For this review, use the dimensioned drawing (mm, ordinates from the lowest corner) and the shaded views. A direction names the side the tool comes from. Coordinates: 2 decimals unless noted, no trailing zeros. Order: outer loops, then holes, each group sorted by start corner. A loop starts at its lowest first (then second) coordinate and runs counter-clockwise, first axis right, second up. Notation, with made-up numbers: M 1,-10.5 L 28,-10.5 A23 cw 28,5.5 Z; hole C 71.25,70 d4. An arc over 180 degrees is marked long. Answer in a Markdown table with one row per item.
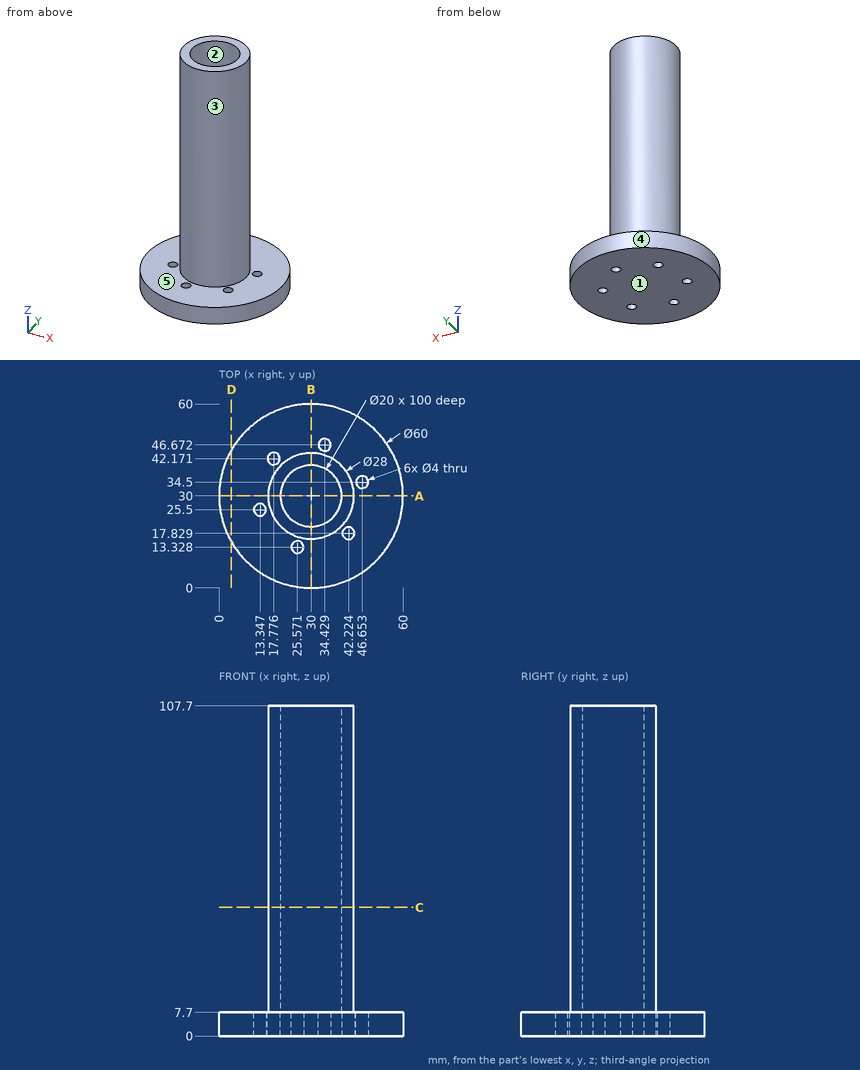
(1) Take a section at D-D (x = 4). Write out the cut boundary in (y, z).
Report:
| item | result |
|---|---|
| outline | M 15.03,0 L 44.97,0 L 44.97,7.7 L 15.03,7.7 Z |
(2) Insertion check: P1, Ø4, axis at x = 40, z = 19, coming from the -Y side; P2, Ø3, axis at x = 48.5, y = 27, coming from the +Z side; P3, Ø22, axis at x = 33.5, y = 28.5, coming from the +Z side; P4, Ø2.5, axis at x = 17.78, y = 42.17, coming from the +Z side. Each pin has a flat end and moves straight along its axis. Give the tip position at first contact, or say it passes through.
Report:
| item | result |
|---|---|
| P1 | y = 18.51 |
| P2 | z = 7.7 |
| P3 | z = 107.7 |
| P4 | through |
(3) To check wall thickness, follow line 1 (Y direction, x = 30, z = 57.5); line 2 (Z direction, x = 5.5, y = 29); line 3 (X direction, y = 33.5, z = 24) (1 decimal). State the ranges of each line that lie inside material, in increasing order. Write a range as [from, to].
Report:
| item | result |
|---|---|
| line 1 | [16, 20], [40, 44] |
| line 2 | [0, 7.7] |
| line 3 | [16.4, 20.6], [39.4, 43.6] |
(4) Take a section at A-A (y = 30). Write out the cut boundary in (x, z), then the cut area to 3 significant figures.
Report:
| item | result |
|---|---|
| outline | M 0,0 L 60,0 L 60,7.7 L 44,7.7 L 44,107.7 L 40,107.7 L 40,7.7 L 20,7.7 L 20,107.7 L 16,107.7 L 16,7.7 L 0,7.7 Z |
| area | 1,260 mm^2 |
(5) The part is to be moulded in two halves that separate along X. For the marked faces 1, 2 and 3, say which applies: +X half, -X half, draft (parallel to the pull), parting line (faces both ways), or undercut.
Report:
| item | result |
|---|---|
| face 1 | draft |
| face 2 | undercut |
| face 3 | parting line |
(6) Take a section at C-C (z = 42). Write out the cut boundary in (x, y).
Report:
| item | result |
|---|---|
| outline | C 30,30 d28; hole C 30,30 d20 |
(7) Machinability: for the marked faces 4 and 5, which of the approach directions +Z, -Z, +X, -X, +Y, -Y give a long, thin tool a straight path to every point of the face, cutting with its end or side? Answer none if there is none.
Report:
| item | result |
|---|---|
| face 4 | +Z, -Z |
| face 5 | +Z |
